from build123d import *

# Parameters (mm, degrees)
SKETCH1_R           = 57.15
BOSS_EXTRUDE5_DEPTH = 25.4
SKETCH4_R           = 25.4
BOSS_EXTRUDE7_DEPTH = 12.7
SKETCH5_W           = 9.525
SKETCH5_H           = 56.448043325
BOSS_EXTRUDE8_DEPTH = 22.225


with BuildPart() as part:
    # Sketch1 → Boss-Extrude5 (new body)
    with BuildSketch(Plane.XY):
        Circle(SKETCH1_R)
        with BuildLine():
            Line((-4.7625, -18.279615818), (-4.7625, -13.517115818))
            Line((-4.7625, -13.517115818), (4.7625, -13.517115818))
            Line((4.7625, -13.517115818), (4.7625, -18.279615818))
            ThreePointArc((4.7625, -18.279615818), (0, -46.0375), (-4.7625, -18.279615818))
        make_face(mode=Mode.SUBTRACT)
        with BuildLine():
            ThreePointArc((-25.069578471, -27.666345352), (-32.776314377, -30.426898024), (-39.77908045, -26.187122475))
            ThreePointArc((-39.77908045, -26.187122475), (-45.621372905, -13.668612193), (-47.625, 0))
            ThreePointArc((-47.625, 0), (0, 47.625), (47.625, 0))
            ThreePointArc((47.625, 0), (45.621372905, -13.668612193), (39.77908045, -26.187122475))
            ThreePointArc((39.77908045, -26.187122475), (32.776314377, -30.426898024), (25.069578471, -27.666345352))
            ThreePointArc((25.069578471, -27.666345352), (0, -6.35), (-25.069578471, -27.666345352))
        make_face(mode=Mode.SUBTRACT)
    extrude(amount=BOSS_EXTRUDE5_DEPTH)

    # Sketch4 → Boss-Extrude7 (add)
    with BuildSketch(Plane.XY.offset(25.4)):
        with Locations(Location((0, -31.75, 0), (0, 0, 170.748186525))):
            Circle(SKETCH4_R)
        with BuildLine():
            Line((-4.7625, -18.279615818), (-4.7625, -13.517115818))
            Line((-4.7625, -13.517115818), (4.7625, -13.517115818))
            Line((4.7625, -13.517115818), (4.7625, -18.279615818))
            ThreePointArc((4.7625, -18.279615818), (0, -46.0375), (-4.7625, -18.279615818))
        make_face(mode=Mode.SUBTRACT)
    extrude(amount=BOSS_EXTRUDE7_DEPTH)

    # Sketch5 → Boss-Extrude8 (add)
    with BuildSketch(Plane.XY):
        with Locations((0, 20.552658513)):
            Rectangle(SKETCH5_W, SKETCH5_H)
    extrude(amount=BOSS_EXTRUDE8_DEPTH)


solid = part.part
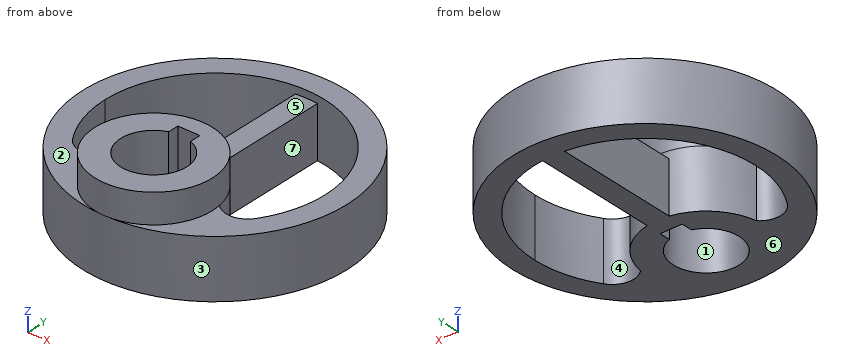
Can you work these out from the model? Positions are in its coordinate system, mm. Face numbers are marked on the shaded views. A direction names the side the tool comes from. Coordinates: 2 decimals unless noted, no trailing zeros. Write each loop counter-clockwise with the first axis right and the second up, starting at its lowest first coordinate (ties: lowest second). Pieces come first, ordered by that corner, then holes.
Q1. If we mould it in two halves opening along X, with no side actions, what happens to the marked faces 1, 2, 3 and 4? For each: +X half, -X half, draft (parallel to the pull), parting line (faces both ways), or undercut.
Results found:
face 1: undercut
face 2: draft
face 3: parting line
face 4: undercut
Q2. Imagine slicing it at B-B, the plane y = 21. List the corners of the cut face in (x, z) for me (1 decimal).
Results found:
outline: (-53.2, 0) - (-42.7, 0) - (-42.7, 25.4) - (-53.2, 25.4) - close; (-4.8, 0) - (4.8, 0) - (4.8, 22.2) - (-4.8, 22.2) - close; (42.7, 0) - (53.2, 0) - (53.2, 25.4) - (42.7, 25.4) - close
Q3. Imagine slicing it at C-C, the plane x = -32. List the corners of the cut face in (y, z) for me.
Results found:
outline: (-47.35, 0) - (-30.47, 0) - (-30.47, 25.4) - (-47.35, 25.4) - close; (35.27, 0) - (47.35, 0) - (47.35, 25.4) - (35.27, 25.4) - close
Q4. Please list where these lines run through material, in increasing order: L1, parallel to Y at x = 0, z = 30; L2, parallel to Y at x = 0, z = 13.5; L3, parallel to Y at x = -6, z = 7.5.
Results found:
L1: y = -57.15 to -46.04, -13.52 to -6.35
L2: y = -57.15 to -46.04, -13.52 to 57.15
L3: y = -56.83 to -44.72, -18.78 to -7.07, 47.25 to 56.83
Q5. Imagine slicing it at A-A, the plane z = 17. Count the separate pieces of the cut face and the enclosed holes in it, plus the area to 3 significant figures.
Results found:
separate pieces: 1
enclosed holes: 3
area: 4,810 mm2
Q6. Which directions (+Z, -Z, +X, -X, +Y, -Y) give clear straight access to the entire face, cutting with the end or side of a thin tool? Please do the marked faces 5, 6 and 7.
Results found:
face 5: +Z
face 6: -Z, +X, -X, +Y, -Y
face 7: +Z, -Z
Q7. For P1, Ø5, axis at y = -17, z = 14.5, coming from the -X side; P2, Ø3, axis at x = 0, z = 15.5, coming from the -Y side; P3, Ø11, axis at y = 17, z = 14.5, coming from the -X side, each with a flat end and sliding along its axis, tell me the tip position at first contact or that it passes through.
Results found:
P1: stops at x = -55.28
P2: stops at y = -57.15
P3: stops at x = -55.98
